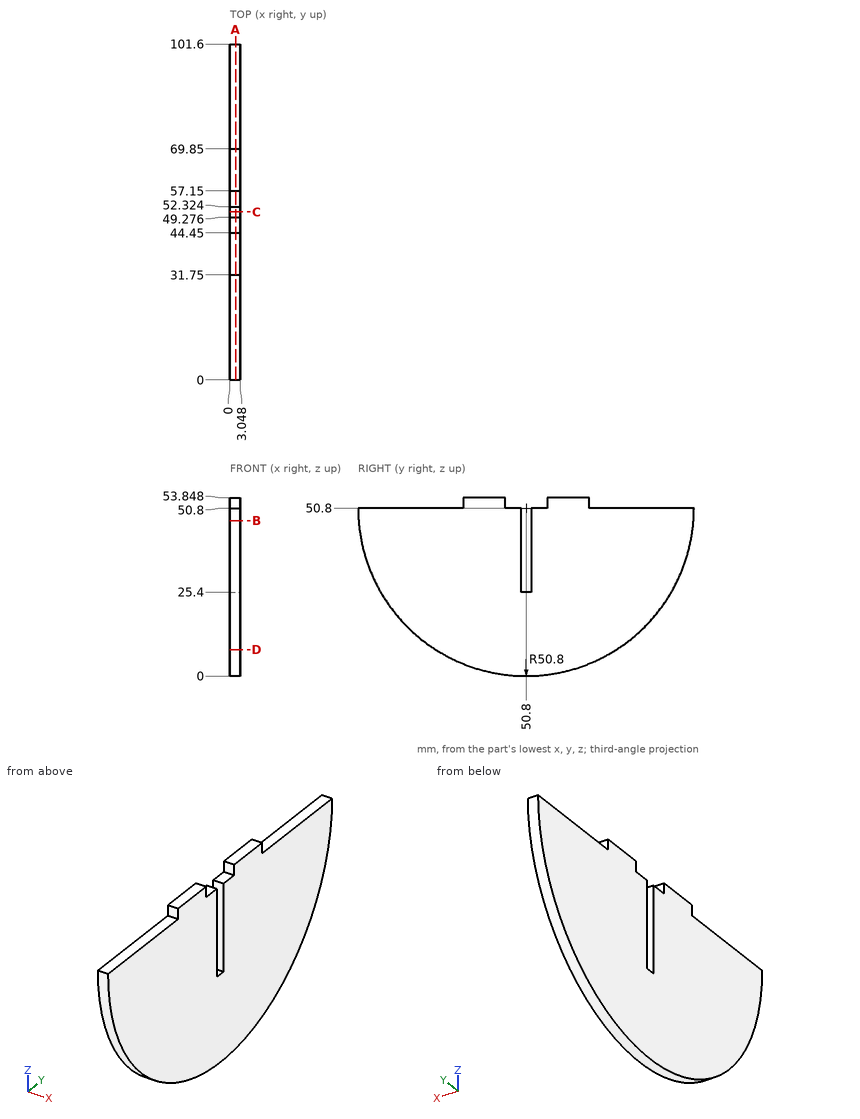
Answer from the drawing. Dimensions are ordinates in mm from the lowest x, y and z of the part. Round coordinates to 2 decimals unless told otherwise and drop trailing zeros. Write each loop counter-clockwise with the first axis right and the second up, starting at its lowest first coordinate (ties: lowest second). Pieces come first, ordered by that corner, then holes. Notation, with made-up numbers: (86, 11.5) -> (143, 11.5) arc R29 cw to (143, 33.5) -> close; hole circle Ø5 at (49, 71.25). An arc over 180 degrees is marked (long way). Answer in a Markdown table with one row per item. Add a question column.
1) Find section B-B, the plane z = 47. Determine the outline of the cut face in (x, y), and give its area (3 significant figures).
2) Find section D-D, the plane z = 8. Determine the outline of the cut face in (x, y), and give its area (3 significant figures).
3) Find section A-A, the plane x = 1.7. Determine the outline of the cut face in (y, z).
4) Consider line 1 (Y direction, x = 2.15, z = 51.5); line 2 (Y direction, x = 2.45, z = 47); line 3 (Z direction, x = 0.85, y = 52.5). Determine where each line is inside the solid, lowest interval first.
5) Given P1, Ø0.9, axis at x = 1, z = 51.5, coming from the +Y side; P2, Ø0.9, axis at x = 1.5, z = 38.5, coming from the +Y side; P3, Ø0.9, axis at x = 2, y = 50, coming from the +Z side, each flat-ended and moving along its own axis, determine where each tip first touches the part or whether it passes through.
6) Find section C-C, the plane y = 50.8. Determine the outline of the cut face in (x, z), and give its area (3 significant figures).
Findings below:
| question | item | result |
|---|---|---|
| 1 | outline | (0, 0.14) -> (3.05, 0.14) -> (3.05, 49.28) -> (0, 49.28) -> close; (0, 52.32) -> (3.05, 52.32) -> (3.05, 101.46) -> (0, 101.46) -> close |
| 1 | area | 300 mm² |
| 2 | outline | (0, 23.44) -> (3.05, 23.44) -> (3.05, 78.16) -> (0, 78.16) -> close |
| 2 | area | 167 mm² |
| 3 | outline | (0, 50.8) arc R50.8 ccw to (101.6, 50.8) -> (69.85, 50.8) -> (69.85, 53.85) -> (57.15, 53.85) -> (57.15, 50.8) -> (52.32, 50.8) -> (52.32, 25.4) -> (49.28, 25.4) -> (49.28, 50.8) -> (44.45, 50.8) -> (44.45, 53.85) -> (31.75, 53.85) -> (31.75, 50.8) -> close |
| 4 | line 1 | 31.75 to 44.45, 57.15 to 69.85 |
| 4 | line 2 | 0.14 to 49.28, 52.32 to 101.46 |
| 4 | line 3 | 0.03 to 50.8 |
| 5 | P1 | y = 69.85 |
| 5 | P2 | y = 100.2 |
| 5 | P3 | z = 25.4 |
| 6 | outline | (0, 0) -> (3.05, 0) -> (3.05, 25.4) -> (0, 25.4) -> close |
| 6 | area | 77.4 mm² |
